Design review of the part built by this model. Coordinates are the model's own, in mm. Face numbers are marked on the shaded views. A direction names the side the tool comes from. Coordinates: 2 decimals unless noted, no trailing zeros. Loops run counter-clockwise (first coordinate to the right, second up) from the corner with the lowest first, then second, coordinate; pieces in that order, holes last.
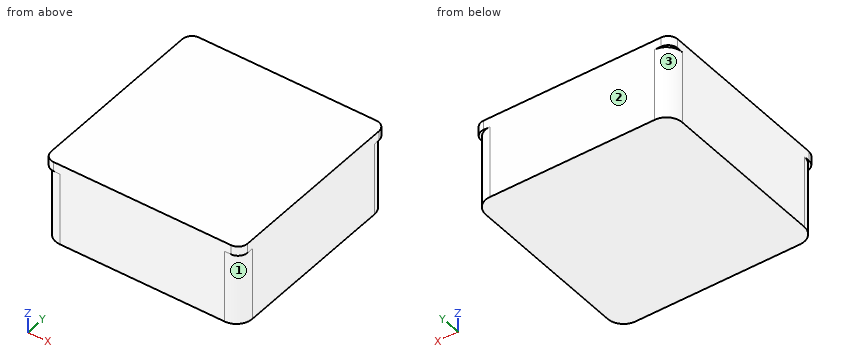
Autodesk Fusion 360 part; units mm, degrees
sketch "Sketch1" plane through (0, 0, 0) normal (0, 0, 1) x (1, 0, 0)
  line L0 (155, 155) -> (-155, 155)
  line L1 (-155, 155) -> (-155, -155)
  line L2 (-155, -155) -> (155, -155)
  line L3 (155, -155) -> (155, 155)
  line L4 (155, 155) -> (-155, -155) construction
  line L5 (-155, 155) -> (155, -155) construction
  dimension "d1" = 310
  dimension "d2" = 310
extrude "Extrude1" add sketch "Sketch1" along normal blind 115
shell "Shell1" thickness 10 removed faces 1 at (-51.6667, 51.6667, 115)
fillet "Fillet1" radius 25 4 edges at (-155, -155, 57.5) (155, -155, 57.5) (-155, 155, 57.5) (155, 155, 57.5)
ref_plane "WorkPlane1" through (0, 0, 115) normal (0, 0, 1) x (1, 0, 0)
sketch "Sketch2" plane through (0, 0, 115) normal (0, 0, 1) x (1, 0, 0)
  line L0 (155, 155) -> (-155, 155)
  line L1 (-155, 155) -> (-155, -155)
  line L2 (-155, -155) -> (155, -155)
  line L3 (155, -155) -> (155, 155)
  line L4 (155, 155) -> (-155, -155) construction
  line L5 (-155, 155) -> (155, -155) construction
  line L6 (-145, 145) -> (145, 145)
  line L7 (145, 145) -> (145, -145)
  line L8 (145, -145) -> (-145, -145)
  line L9 (-145, -145) -> (-145, 145)
  line L10 (-145, 145) -> (145, -145) construction
  line L11 (145, 145) -> (-145, -145) construction
  dimension "d9" = 310
  dimension "d10" = 310
  dimension "d11" = 290
  dimension "d12" = 290
extrude "Extrude2" add sketch "Sketch2" against normal blind 15 contours L6 L7 L8 L9
extrude "Extrude3" add sketch "Sketch2" along normal blind 15 contours L0 L1 L2 L3 | L6 L7 L8 L9
fillet "Fillet2" radius 15 4 edges at (-155, 155, 122.5) (-155, -155, 122.5) (155, -155, 122.5) (155, 155, 122.5)
Q1. Take a section at B-B, the plane y = 55. Write out the cut boundary in (x, z), then the cut area to 3 significant figures.
Q2. Machinability: for the marked faces 1, 2 and 3, which of the approach directions +Z, -Z, +X, -X, +Y, -Y give a long, thin tool a straight path to every point of the face, cutting with its end or side? Answer none if there is none.
Q3. Take a section at A-A, the plane z = 76. Write out the cut boundary in (x, y).
Q4. For line 1 (Z direction, x = -72, y = 84); line 2 (X direction, y = -64.5, z = 69), list the stretches that pass through material, from the lowest coordinate up.
Entries:
1. outline: (-155, 0) - (155, 0) - (155, 130) - (-155, 130) - close; hole (-145, 10) - (145, 10) - (145, 100) - (-145, 100) - close
1. area: 14,200 mm2
2. face 1: -Z, +X, -Y
2. face 2: +Z, -Z, +X, -X, +Y
2. face 3: -Z, -X, +Y
3. outline: (-155, -130) arc R25 ccw to (-130, -155) - (130, -155) arc R25 ccw to (155, -130) - (155, 130) arc R25 ccw to (130, 155) - (-130, 155) arc R25 ccw to (-155, 130) - close; hole (-145, -145) - (145, -145) - (145, 145) - (-145, 145) - close
4. line 1: z = 0 to 10, 100 to 130
4. line 2: x = -155 to -145, 145 to 155
